from build123d import *

# Parameters (mm, degrees)
SKETCH_1_W      = 20
SKETCH_1_H      = 5
EXTRUDE_1_DEPTH = 35
SKETCH_2_W      = 30
SKETCH_2_H      = 20
EXTRUDE_2_DEPTH = 3
FILLET_1_R      = 2
FILLET_2_R      = 2
FILLET_3_R      = 2
FILLET_4_R      = 2
SKETCH_4_W      = 30
SKETCH_4_H      = 40
EXTRUDE_3_DEPTH = 2.5
FILLET_5_R      = 2
FILLET_6_R      = 2


with BuildPart() as part:
    # 草图1 → 凸台-拉伸1 (new body)
    with BuildSketch(Plane(origin=(0, 0, 0), x_dir=(0, 0, -1), z_dir=(1, 0, 0))):
        Rectangle(SKETCH_1_W, SKETCH_1_H)
    extrude(amount=-EXTRUDE_1_DEPTH)

    # 草图2 → 凸台-拉伸2 (add)
    with BuildSketch(Plane(origin=(0, 0, 0), x_dir=(0, 0, -1), z_dir=(1, 0, 0))):
        Rectangle(SKETCH_2_W, SKETCH_2_H)
    extrude(amount=EXTRUDE_2_DEPTH)

    # 圆角1
    fillet_1_edges = [part.edges().sort_by_distance(p)[0] for p in [
        (1.5, 10, -15),
    ]]
    fillet(fillet_1_edges, radius=FILLET_1_R)

    # 圆角2
    fillet_2_edges = [part.edges().sort_by_distance(p)[0] for p in [
        (1.5, 10, 15),
    ]]
    fillet(fillet_2_edges, radius=FILLET_2_R)

    # 圆角3
    fillet_3_edges = [part.edges().sort_by_distance(p)[0] for p in [
        (1.5, -10, -15),
    ]]
    fillet(fillet_3_edges, radius=FILLET_3_R)

    # 圆角4
    fillet_4_edges = [part.edges().sort_by_distance(p)[0] for p in [
        (1.5, -10, 15),
    ]]
    fillet(fillet_4_edges, radius=FILLET_4_R)

    # 草图4 → 凸台-拉伸3 (add, symmetric)
    with BuildSketch(Plane(origin=(0, 0, 0), x_dir=(1, 0, 0), z_dir=(0, 1, 0))):
        with Locations((-20, 0)):
            Rectangle(SKETCH_4_W, SKETCH_4_H)
    extrude(amount=EXTRUDE_3_DEPTH, both=True)

    # 圆角5
    fillet_5_edges = [part.edges().sort_by_distance(p)[0] for p in [
        (-5, 0, -10),
    ]]
    fillet(fillet_5_edges, radius=FILLET_5_R)

    # 圆角6
    fillet_6_edges = [part.edges().sort_by_distance(p)[0] for p in [
        (-5, 0, 10),
    ]]
    fillet(fillet_6_edges, radius=FILLET_6_R)


solid = part.part
Design review of the part built by this model. Coordinates are the model's own, in mm. A direction names the side the tool comes from. Coordinates: 2 decimals unless noted, no trailing zeros. Loops run counter-clockwise (first coordinate to the right, second up) from the corner with the lowest first, then second, coordinate; pieces in that order, holes last. Notation, with made-up numbers: (2, 46) -> (16, 46) arc R21 ccw to (16, 62) -> close; hole circle Ø7 at (27, 58.25). An arc over 180 degrees is marked (long way). Use a Markdown table: item, result. Add a question column.
Item 1: We need section D-D, the plane x = -8.5. Write out the cut boundary in (y, z), and give its area (3 significant figures).
Item 2: We need section A-A, the plane z = -11. Write out the cut boundary in (x, y).
Item 3: Machinability: for faces 1 (the flat face through (1, 0, 15)), 2 (the flat face through (-5, 0, 16)), 3 (the flat face through (1, 0, -15)), 4 (the flat face through (-18, -2.5, 0)), which of the approach directions +Z, -Z, +X, -X, +Y, -Y give a long, thin tool a straight path to every point of the face, cutting with its end or side? Answer none if there is none.
Item 4: Clearance check with flat-ended pins moving along their axes: P1, Ø5, axis at x = -28.5, z = 7.5, coming from the +Y side; P2, Ø2.5, axis at y = 0, z = -17, coming from the +X side; P3, Ø3, axis at y = 5, z = 10.5, coming from the -X side. State where each tip first meets the part, or that it passes through.
Item 5: We need section B-B, the plane y = 0. Write out the cut boundary in (x, z), and give its area (3 significant figures).
Item 6: The part is to be moulded in two halves that separate along X. For faces 5 (the flat face through (-18, 2.5, 0)), 6 (the flat face through (3, 0, 0)), 7 (the flat face through (0, 5, 0)), 8 (the flat face through (-5, 0, -16)), say which applies: +X half, -X half, draft (parallel to the pull), parting line (faces both ways), or undercut.
Item 7: We need section C-C, the plane z = -7. Write out the cut boundary in (x, y), and give its area (3 significant figures).
Item 8: Wall thickness on L1, parallel to X at y = -1, z = 12; L2, parallel to Y at x = -9, z = 3; L3, parallel to X at y = -5, z = 12: over which ranges is each line inside the solid? List them lowest first. Write a range as from..to.
Numbers:
| question | item | result |
|---|---|---|
| 1 | outline | (-2.5, -20) -> (2.5, -20) -> (2.5, 20) -> (-2.5, 20) -> close |
| 1 | area | 200 mm^2 |
| 2 | outline | (-35, -2.5) -> (-4.73, -2.5) -> (-4.73, 2.5) -> (-35, 2.5) -> close; (0, -10) -> (3, -10) -> (3, 10) -> (0, 10) -> close |
| 3 | face 1 | +Z, +X, +Y, -Y |
| 3 | face 2 | +Z, +Y, -Y |
| 3 | face 3 | -Z, +X, +Y, -Y |
| 3 | face 4 | +Z, -Z, -X, -Y |
| 4 | P1 | stops at y = 2.5 |
| 4 | P2 | stops at x = -5 |
| 4 | P3 | stops at x = 0 |
| 5 | outline | (-35, -20) -> (-5, -20) -> (-5, -12) arc R2 cw to (-3, -10) -> (0, -10) -> (0, -15) -> (3, -15) -> (3, 15) -> (0, 15) -> (0, 10) -> (-3, 10) arc R2 cw to (-5, 12) -> (-5, 20) -> (-35, 20) -> close |
| 5 | area | 1,390 mm^2 |
| 6 | face 5 | draft |
| 6 | face 6 | +X half |
| 6 | face 7 | undercut |
| 6 | face 8 | undercut |
| 7 | outline | (-35, -2.5) -> (0, -2.5) -> (0, -10) -> (3, -10) -> (3, 10) -> (0, 10) -> (0, 2.5) -> (-35, 2.5) -> close |
| 7 | area | 235 mm^2 |
| 8 | L1 | x = -35..-5, 0..3 |
| 8 | L2 | y = -2.5..2.5 |
| 8 | L3 | x = 0..3 |
